Autodesk Inventor part; units mm, degrees
ref_plane "YZ Plane" through (0, 0, 0) normal (1, 0, 0) x (0, 1, 0)
ref_plane "XZ Plane" through (0, 0, 0) normal (0, 1, 0) x (-1, 0, 0)
ref_plane "XY Plane" through (0, 0, 0) normal (0, 0, 1) x (1, 0, 0)
sketch "Skizze1" plane through (0, 0, 0) normal (0, 0, 1) x (1, 0, 0)
  line L0 (-20, 0) -> (20, 0) construction
  line L1 (-20, -8) -> (20, -8)
  line L2 (20, 8) -> (-20, 8)
  arc A0 (-20, 8) -> (-20, -8) centre (-20, 0) ccw
  arc A1 (20, -8) -> (20, 8) centre (20, 0) ccw
  line L3 (-25, 0) -> (25, 0) construction
  line L4 (-25, -14) -> (25, -14)
  line L5 (25, 14) -> (-25, 14)
  arc A2 (-25, 14) -> (-25, -14) centre (-25, 0) ccw
  arc A3 (25, -14) -> (25, 14) centre (25, 0) ccw
  point P0 (0, 0)
  dimension "d0" = 16
  dimension "d1" = 40
  dimension "d2" = 28
  dimension "d3" = 50
extrude "Extrusion1" add sketch "Skizze1" along normal blind 14 contours A0 L2 A1 L1
extrude "Extrusion2" add sketch "Skizze1" against normal blind 33.623 contours A0 L2 A1 L1 | A2 L5 A3 L4
equation "\"Height\" = 47.623"
properties part number "Gabel_DistanzStopper"
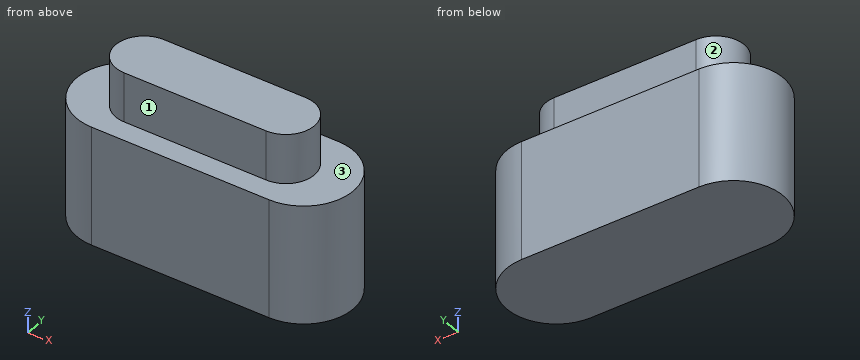
Can you work these out from the model? Positions are in its coordinate system, mm. Face numbers are marked on the shaded views. A direction names the side the tool comes from. Round coordinates to 2 decimals unless told otherwise and drop trailing zeros. Loops run counter-clockwise (first coordinate to the right, second up) from the corner with the lowest first, then second, coordinate; pieces in that order, holes last. Notation, with made-up numbers: M 20,6 L 58,6 A19 ccw 58,16 Z; hole C 71,79.25 d1. An arc over 180 degrees is marked long. Answer in a Markdown table with one row per item.
1. If we section it at B-B, the plane y = -3.5: Please give me the cut outline in (x, z), plus the area to 3 significant figures.
Established:
| item | result |
|---|---|
| outline | M -38.56,-33.62 L 38.56,-33.62 L 38.56,0 L 27.19,0 L 27.19,14 L -27.19,14 L -27.19,0 L -38.56,0 Z |
| area | 3,350 mm² |
2. On a 3-axis mill with a long thin cutter (end or side, diameter ignored), from which of +Z, -Z, +X, -X, +Y, -Y can I reach the whole of each face in a straight line? I mean the marked faces 1, 2 and 3. Say none if no direction works.
Established:
| item | result |
|---|---|
| face 1 | +Z, +X, -X, -Y |
| face 2 | +Z, -X |
| face 3 | +Z |
3. Please list where these lines run through material, in increasing order: line 1 (Z direction, x = -14, y = -13); line 2 (X direction, y = -0.5, z = -3); line 3 (Y direction, x = -20.5, z = 4). Write a range as from..to.
Established:
| item | result |
|---|---|
| line 1 | -33.62..0 |
| line 2 | -38.99..38.99 |
| line 3 | -7.98..7.98 |
4. If we section it at A-A, the plane x = -2: Please give me the cut outline in (y, z), plus the area to 3 significant figures.
Established:
| item | result |
|---|---|
| outline | M -14,-33.62 L 14,-33.62 L 14,0 L 8,0 L 8,14 L -8,14 L -8,0 L -14,0 Z |
| area | 1,170 mm² |
5. I'm going to push flat-ended pins straight in: pin 1 Ø8 at (y, z) = (-10.5, -9) entering from -X; pin 2 Ø1.5 at (y, z) = (4, -9.5) entering from -X; pin 3 Ø7 at (x, z) = (-1, 10.5) entering from -Y. Where does each tip first touch, or does it pass through?
Established:
| item | result |
|---|---|
| pin 1 | x = -37.4 |
| pin 2 | x = -38.62 |
| pin 3 | y = -8 |
6. If we section it at D-D, the plane x = -33: Please give me the cut outline in (y, z).
Established:
| item | result |
|---|---|
| outline | M -11.49,-33.62 L 11.49,-33.62 L 11.49,0 L -11.49,0 Z |
7. If we section it at C-C, the plane z = -1: Please give me the cut outline in (x, y).
Established:
| item | result |
|---|---|
| outline | M -25,-14 L 25,-14 A14 ccw 25,14 L -25,14 A14 ccw Z |
